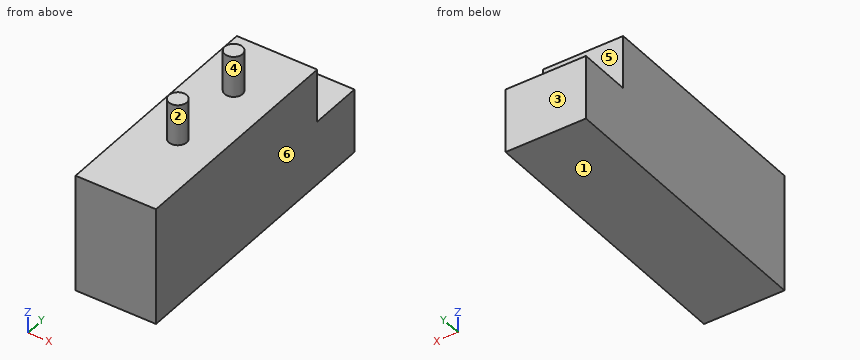
Autodesk Inventor part; units mm, degrees
ref_plane "YZ Plane" through (0, 0, 0) normal (1, 0, 0) x (0, 1, 0)
ref_plane "XZ Plane" through (0, 0, 0) normal (0, 1, 0) x (-1, 0, 0)
ref_plane "XY Plane" through (0, 0, 0) normal (0, 0, 1) x (1, 0, 0)
sketch "Sketch1" plane through (0, 0, 0) normal (0, 0, 1) x (1, 0, 0)
  line L0 (0, 112) -> (0, -112) construction
  line L1 (-31.5, 0) -> (31.5, 0) construction
  line L2 (-22.5, 80) -> (22.5, 80)
  line L3 (22.5, 80) -> (22.5, -80)
  line L4 (22.5, -80) -> (-22.5, -80)
  line L5 (-22.5, -80) -> (-22.5, 80)
  line L6 (-22.5, 80) -> (22.5, -80) construction
  line L7 (22.5, 80) -> (-22.5, -80) construction
  point P0 (0, 0)
  dimension "d4" = 160
  dimension "d5" = 45
extrude "Extrusion3" add sketch "Sketch1" along normal blind 66
sketch "Sketch2" plane through (0, 0, 66) normal (0, 0, 1) x (1, 0, 0)
  circle A0 centre (0, -30) radius 5
  circle A1 centre (0, 15) radius 5
  line L0 (-22.5, -80) -> (22.5, -80)
  point P0 (0, 0)
  dimension "d8" = 10
  dimension "d9" = 50
  dimension "d10" = 45
extrude "Extrusion4" add sketch "Sketch2" along normal blind 23
thread "Thread1"
thread "Thread2"
sketch "Sketch3" plane through (22.5, -80, 0) normal (1, 0, 0) x (0, 0, -1)
  line L0 (0, 160) -> (0, 0)
  line L1 (0, 160) -> (-66, 160)
  line L2 (-66, 0) -> (-66, 160)
  line L3 (0, 0) -> (-66, 0)
  line L4 (-66, 160) -> (-36, 160)
  line L5 (-36, 160) -> (-36, 130)
  line L6 (-36, 130) -> (-66, 130)
  line L7 (-66, 130) -> (-66, 160)
  point P0 (0, 80)
  dimension "d17" = 30
  dimension "d18" = 30
extrude "Extrusion5" cut sketch "Sketch3" against normal through all contours L5 L6 L2 L1
properties part number "17-0028-0082"
Geometry: final body of the model. Coordinates: model frame, mm. Face numbers are marked on the shaded views. A direction names the side the tool comes from. Coordinates: 2 decimals unless noted, no trailing zeros. Loops run counter-clockwise (first coordinate to the right, second up) from the corner with the lowest first, then second, coordinate; pieces in that order, holes last. Notation, with made-up numbers: M 48.25,24.5 L 60.25,24.5 A26 ccw 60.25,50.5 Z; hole C -2,54 d5. An arc over 180 degrees is marked long. One line per item, written item: value. Start each with the question number.
1) Material intervals for L1, parallel to Y at x = 6.5, z = 55; L2, parallel to Z at x = 16.5, y = 36; L3, parallel to X at y = -26.5, z = 72.5, sorted ascending. Write a range as from..to.
2) Reachability of the marked faces 5 and 6 from +Z, -Z, +X, -X, +Y, -Y: full face, straight path, thin tool, end or side. Return the list, or none.
3) Cut plane C-C (z = 41). Return loops of the section in (x, y).
4) Draft query along Y for the marked faces 1, 2, 3 and 4. Return one class per face: released by +Y, released by -Y, zero draft, split by the parting line, or undercut.
5) Cut plane D-D (x = -12). Return loops of the section in (y, z), then the cut area to 3 significant figures.
6) Pin query (flat end, axial travel): P1, Ø6, axis at x = -14, z = 59.5, coming from the +Y side; P2, Ø10, axis at x = -9.5, y = -36.5, coming from the -Z side; P3, Ø3, axis at x = 11.5, y = 26.5, coming from the +Z side; P4, Ø15, axis at x = -10, y = 71, coming from the +Z side. Return the tip coordinate at first contact, or that it passes through.
7) Cut plane B-B (y = -30). Return loops of the section in (x, z).
8) Cut plane A-A (x = 0). Return loops of the section in (y, z).
Evaluation:
1. L1: -80..50
1. L2: 0..66
1. L3: -3.57..3.57
2. face 5: +Z, +X, -X, +Y
2. face 6: +Z, -Z, +X, +Y, -Y
3. outline: M -22.5,-80 L 22.5,-80 L 22.5,50 L -22.5,50 Z
4. face 1: zero draft
4. face 2: undercut
4. face 3: released by +Y
4. face 4: undercut
5. outline: M -80,0 L 80,0 L 80,36 L 50,36 L 50,66 L -80,66 Z
5. area: 9,660 mm^2
6. P1: y = 50
6. P2: z = 0
6. P3: z = 66
6. P4: z = 36
7. outline: M -22.5,0 L 22.5,0 L 22.5,66 L 5,66 L 5,89 L -5,89 L -5,66 L -22.5,66 Z
8. outline: M -80,0 L 80,0 L 80,36 L 50,36 L 50,66 L 20,66 L 20,89 L 10,89 L 10,66 L -25,66 L -25,89 L -35,89 L -35,66 L -80,66 Z
